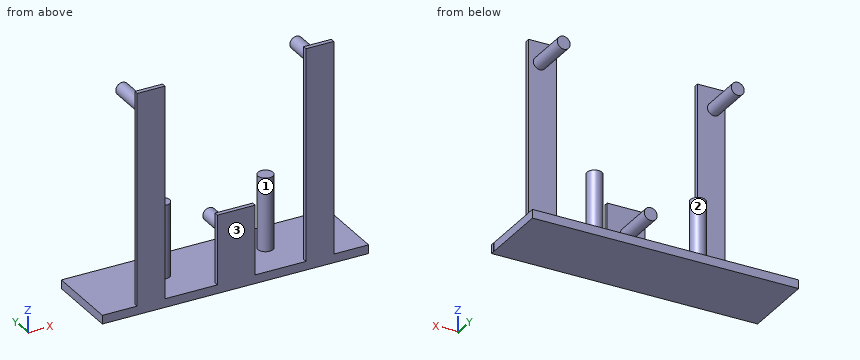
```python
from build123d import *

# Parameters (mm, degrees)
BOSS_EXTRUDE1_START = 5.08
SKETCH1_R           = 4.445
BOSS_EXTRUDE1_DEPTH = 43.18
SKETCH2_W           = 156.929873994
SKETCH2_H           = 41.148
BOSS_EXTRUDE2_DEPTH = 5.08
SKETCH3_W           = 22.259444318
SKETCH3_H           = 46.05258329
BOSS_EXTRUDE3_DEPTH = 2.54
SKETCH4_W           = 16.338838854
SKETCH4_H           = 129.983858652
BOSS_EXTRUDE4_DEPTH = 2.54
SKETCH5_W           = 156.97130624
SKETCH5_H           = 5.08
BOSS_EXTRUDE5_DEPTH = 2.54
SKETCH6_R           = 3.81
BOSS_EXTRUDE6_DEPTH = 25.4
SKETCH8_R           = 3.81
BOSS_EXTRUDE7_DEPTH = 25.4


with BuildPart() as part:
    # Sketch1 → Boss-Extrude1 (new body)
    with BuildSketch(Plane.XY.offset(BOSS_EXTRUDE1_START)):
        with Locations((29.969120003, 8.382)):
            Circle(SKETCH1_R)
    extrude(amount=-BOSS_EXTRUDE1_DEPTH)


with BuildPart() as body_2:
    # Mirror2: mirrored copy
    add(part.part.mirror(Plane(origin=(-0.510879997, 0, 0), x_dir=(0, 0, 1), z_dir=(1, 0, 0))))


with BuildPart() as part_1:
    add(part.part)

    add(body_2.part)  # Boss-Extrude2 merges body 2
    # Sketch2 → Boss-Extrude2 (add)
    with BuildSketch(Plane(origin=(0, 0, -38.1), x_dir=(-1, 0, 0), z_dir=(0, 0, -1))):
        with Locations((0.510879997, 8.382)):
            Rectangle(SKETCH2_W, SKETCH2_H)
    extrude(amount=BOSS_EXTRUDE2_DEPTH)

    # Sketch3 → Boss-Extrude3 (add)
    with BuildSketch(Plane.XZ.offset(12.192)):
        with Locations((0, -20.153708355)):
            Rectangle(SKETCH3_W, SKETCH3_H)
    extrude(amount=BOSS_EXTRUDE3_DEPTH)

    # Sketch4 → Boss-Extrude4 (add)
    with BuildSketch(Plane(origin=(0, -12.192, 0), x_dir=(-1, 0, 0), z_dir=(0, -1, 0))):
        with Locations((50.295624604, -21.811929326)):
            Rectangle(SKETCH4_W, SKETCH4_H)
    boss_extrude4 = extrude(amount=BOSS_EXTRUDE4_DEPTH)

    # Mirror3: Boss-Extrude4 across plane
    add(boss_extrude4.mirror(Plane(origin=(-0.510879997, 0, 0), x_dir=(0, 0, 1), z_dir=(1, 0, 0))))

    # Sketch5 → Boss-Extrude5 (add)
    with BuildSketch(Plane.XZ.offset(12.192)):
        with Locations((-0.490163874, -40.64)):
            Rectangle(SKETCH5_W, SKETCH5_H)
    extrude(amount=BOSS_EXTRUDE5_DEPTH)

    # Sketch6 → Boss-Extrude6 (add)
    with BuildSketch(Plane(origin=(0, -12.192, 0), x_dir=(1, 0, 0), z_dir=(0, 1, 0))):
        with Locations(Location((-0.510879997, 12.643336172, 0), (0, 0, 270))):
            Circle(SKETCH6_R)
    extrude(amount=BOSS_EXTRUDE6_DEPTH)

    # Sketch8 → Boss-Extrude7 (add)
    with BuildSketch(Plane(origin=(0, -12.192, 0), x_dir=(1, 0, 0), z_dir=(0, 1, 0))):
        with Locations(Location((50.792572725, -74.463197468, 0), (0, 0, 90))):
            Circle(SKETCH8_R)
    boss_extrude7 = extrude(amount=BOSS_EXTRUDE7_DEPTH)

    # Mirror4: Boss-Extrude7 across plane
    add(boss_extrude7.mirror(Plane(origin=(-0.510879997, 0, 0), x_dir=(0, 0, 1), z_dir=(1, 0, 0))))


solid = part_1.part
```
Part model, mm, in its own coordinate system. Face numbers are marked on the shaded views. Round coordinates to 2 decimals unless told otherwise and drop trailing zeros. Write each loop counter-clockwise with the first axis right and the second up, starting at its lowest first coordinate (ties: lowest second). Pieces come first, ordered by that corner, then holes.
Item 1: Cut at A-A, the plane z = 58.5. Give the cut face in (x, y), plus the area to 3 significant figures.
Results:
outline: (-58.47, -14.73) - (-42.13, -14.73) - (-42.13, -12.19) - (-58.47, -12.19) - close; (41.1, -14.73) - (57.44, -14.73) - (57.44, -12.19) - (41.1, -12.19) - close
area: 83.0 mm2
Item 2: Cut at C-C, the plane y = -8. Give the cut face in (x, z).
Results:
outline: (-78.98, -43.18) - (77.95, -43.18) - (77.95, -38.1) - (-78.98, -38.1) - close; circle Ø7.62 at (-51.81, 74.46); circle Ø7.62 at (-0.51, -12.64); circle Ø7.62 at (50.79, 74.46)
Item 3: Cut at B-B, the plane z = -21.5. Give the cut face in (x, y) (3 decimals).
Results:
outline: (-58.465, -14.732) - (-42.126, -14.732) - (-42.126, -12.192) - (-58.465, -12.192) - close; circle Ø8.89 at (-30.991, 8.382); (-11.13, -14.732) - (11.13, -14.732) - (11.13, -12.192) - (-11.13, -12.192) - close; circle Ø8.89 at (29.969, 8.382); (41.104, -14.732) - (57.443, -14.732) - (57.443, -12.192) - (41.104, -12.192) - close
Item 4: Drop flat-ended pins along their axis: pin 1 Ø6.5 at (x, z) = (-3, -9.5) entering from +Y; pin 2 Ø3 at (y, z) = (-13.5, 18) entering from +X; pin 3 Ø4.5 at (x, y) = (30, 9.5) entering from +Z. Give the stop position or say it passes through.
Results:
pin 1: stops at y = 13.21
pin 2: stops at x = 57.44
pin 3: stops at z = 5.08
Item 5: Cut at D-D, the plane x = 28. Give the cut face in (y, z).
Results:
outline: (-14.73, -43.18) - (28.96, -43.18) - (28.96, -38.1) - (12.37, -38.1) - (12.37, 5.08) - (4.4, 5.08) - (4.4, -38.1) - (-14.73, -38.1) - close
Item 6: Probe L1, parallel to Y at x = 55, z = -12; L2, parallel to Z at x = -37, y = -0.5; L3, parallel to Z at x = -3.5, y = -11. List the from-to ranges inside material, lowest first.
Results:
L1: y = -14.73 to -12.19
L2: z = -43.18 to -38.1
L3: z = -43.18 to -38.1, -15.01 to -10.28
Item 7: Two-plate mould, pull along X, no slides. Class the marked faces 1, 2 and 3: +X half, -X half, draft (parallel to the pull), parting line (faces both ways), or undercut.
Results:
face 1: undercut
face 2: undercut
face 3: draft
